from build123d import *

# Parameters (mm, degrees)
SKETCH1_R           = 100
SKETCH1_R_2         = 25
BOSS_EXTRUDE1_DEPTH = 75
CUT_EXTRUDE1_DEPTH  = 161.078105936
CIRPATTERN1_COUNT   = 20


with BuildPart() as part:
    # Sketch1 → Boss-Extrude1 (new body)
    with BuildSketch(Plane(origin=(0, 0, 0), x_dir=(0, 0, -1), z_dir=(1, 0, 0))):
        Circle(SKETCH1_R)
        Circle(SKETCH1_R_2, mode=Mode.SUBTRACT)
    extrude(amount=BOSS_EXTRUDE1_DEPTH)

    # Sketch2 → Cut-Extrude1 (cut, through all)
    with BuildSketch(Plane(origin=(75, 0, 0), x_dir=(0, 0, -1), z_dir=(1, 0, 0))):
        with BuildLine():
            Line((2.886751346, 99.958324649), (0, 94.958324649))
            Line((0, 94.958324649), (-2.886751346, 99.958324649))
            ThreePointArc((-2.886751346, 99.958324649), (0, 100), (2.886751346, 99.958324649))
        make_face()
    cut_extrude1 = extrude(amount=-CUT_EXTRUDE1_DEPTH, mode=Mode.SUBTRACT)

    # CirPattern1: Cut-Extrude1 ×20 about axis
    cirpattern1_axis = Axis((0, 0, 0), (1, 0, 0))
    for i in range(1, CIRPATTERN1_COUNT):
        add(cut_extrude1.rotate(cirpattern1_axis, i * 360 / CIRPATTERN1_COUNT), mode=Mode.SUBTRACT)


solid = part.part
Part model, mm, in its own coordinate system. Coordinates: 2 decimals unless noted, no trailing zeros. Order: outer loops, then holes, each group sorted by start corner. A loop starts at its lowest first (then second) coordinate and runs counter-clockwise, first axis right, second up. Notation, with made-up numbers: M 46,-31 L 78,-31 A19 ccw 78,-14 Z; hole C 29.5,-26 d9. An arc over 180 degrees is marked long. Use a Markdown table: item, result.
(1) Probe L1, parallel to Z at x = 7, y = 78; L2, parallel to Z at x = 38.5, y = 92.5; L3, parallel to Z at x = 37.5, y = -16. List the from-to ranges inside material, lowest first.
A:
| item | result |
|---|---|
| L1 | z = -62.58 to -58.46, -55.94 to 55.94, 58.46 to 62.58 |
| L2 | z = -38 to -31.78, -28.88 to 28.88, 31.78 to 38 |
| L3 | z = -98.71 to -19.21, 19.21 to 98.71 |
(2) Cut at A-A on y = -13.5. Write the cut outline in (x, z).
A:
| item | result |
|---|---|
| outline | M 0,-99.08 L 75,-99.08 L 75,-21.04 L 0,-21.04 Z; M 0,21.04 L 75,21.04 L 75,99.08 L 0,99.08 Z |
(3) Cut at B-B on z = -65. Write the cut outline in (x, y), then the cut area to 3 significant figures.
A:
| item | result |
|---|---|
| outline | M 0,-75.99 L 75,-75.99 L 75,75.99 L 0,75.99 Z |
| area | 11,400 mm^2 |
(4) Pull direction Z, two halves, no side cores. Call faces 1 (the cylindrical face through (37, -45.2, 89.2)), 2 (the flat face through (38.025, 78.013, -58.489)), 3 (the cylindrical face through (37, 45.2, -89.2)): released by +Z, released by -Z, zero draft, split by the parting line, or undercut.
A:
| item | result |
|---|---|
| face 1 | released by +Z |
| face 2 | undercut |
| face 3 | released by -Z |
(5) Flat gauge pins, fed straight in: pin 1 (4 mm diameter, centred on x = 25.5, z = 29.5, fed in from +Y); pin 2 (8 mm diameter, centred on x = 9, z = 29, fed in from +Y); pin 3 (3 mm diameter, centred on x = 25.5, y = -20.5, fed in from -Z). Where does each tip first touch, or does it go through?
A:
| item | result |
|---|---|
| pin 1 | stops at y = 96.14 |
| pin 2 | stops at y = 96.82 |
| pin 3 | stops at z = -98.18 |
(6) Cut at C-C on y = 71. Write the cut outline in (x, z).
A:
| item | result |
|---|---|
| outline | M 0,-70.42 L 75,-70.42 L 75,70.42 L 0,70.42 Z |
